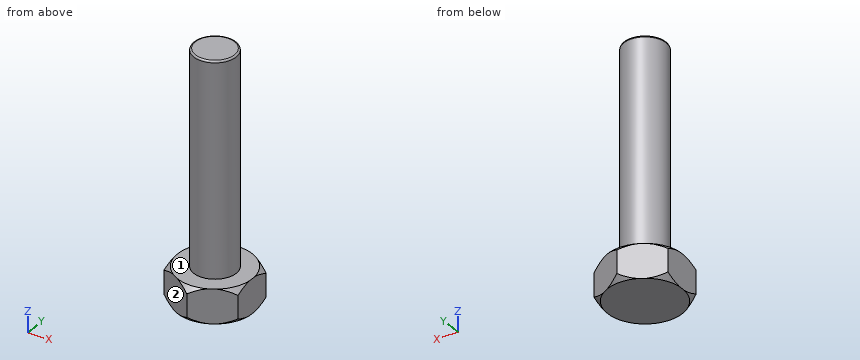
from build123d import *

# Parameters (mm, degrees)
EXTRUDE_1_DEPTH = 3.2
SKETCH_2_R      = 2
EXTRUDE_2_DEPTH = 20
FILLET_1_R      = 0.16


with BuildPart() as part:
    # 草图1 → 凸台-拉伸1 (new body)
    with BuildSketch(Plane.XY):
        Polygon((0, 4.041451884), (-3.5, 2.020725942), (-3.5, -2.020725942), (0, -4.041451884), (3.5, -2.020725942), (3.5, 2.020725942), align=None)
    extrude(amount=-EXTRUDE_1_DEPTH)

    # 草图2 → 凸台-拉伸2 (add)
    with BuildSketch(Plane.XY):
        Circle(SKETCH_2_R)
    extrude(amount=EXTRUDE_2_DEPTH)

    # 圆角1
    fillet_1_edges = [part.edges().sort_by_distance(p)[0] for p in [
        (-2, 0, 20),
    ]]
    fillet(fillet_1_edges, radius=FILLET_1_R)

    # 草图3 → 切除-旋转1 (revolve, cut)
    with BuildSketch(Plane(origin=(0, 0, 0), x_dir=(0, 0, -1), z_dir=(1, 0, 0))):
        Polygon((0.523, 4.041451884), (0, 3.518451884), (0, 4.041451884), align=None)
        Polygon((3.2, 4.041451884), (3.2, 3.518451884), (2.677, 4.041451884), align=None)
    revolve(axis=Axis((0, 0, 0), (0, 0, 1)), mode=Mode.SUBTRACT)


solid = part.part
Verification items for the finished model (mm, model axes). Face numbers are marked on the shaded views. A direction names the side the tool comes from. Coordinates: 2 decimals unless noted, no trailing zeros. Order: outer loops, then holes, each group sorted by start corner. A loop starts at its lowest first (then second) coordinate and runs counter-clockwise, first axis right, second up.
1. Sectioned sample at B-B, the plane z = 9.75. Record the cut outline in (x, y).
Results found:
outline: circle Ø4 at (0, 0)
2. Scan lines: line 1 (Z direction, x = -0.5, y = 2.5); line 2 (Y direction, x = -1.75, z = 19); line 3 (X direction, y = -1.5, z = 14.5). Record each from-to range of solid material in increasing order.
Results found:
line 1: z = -3.2 to 0
line 2: y = -0.97 to 0.97
line 3: x = -1.32 to 1.32
3. Sectioned sample at A-A, the plane y = 0. Record the cut outline in (x, z).
Results found:
outline: (-3.5, -3.2) - (3.5, -3.2) - (3.5, 0) - (2, 0) - (2, 19.84) arc R0.16 ccw to (1.84, 20) - (-1.84, 20) arc R0.16 ccw to (-2, 19.84) - (-2, 0) - (-3.5, 0) - close
4. Go/stop test with flat-tipped pins: pin 1 Ø1.5 at (x, z) = (-1.5, 7) entering from -Y; pin 2 Ø1.5 at (y, z) = (2.5, 15) entering from -X; pin 3 Ø4 at (y, z) = (-1, 2.5) entering from -X. Record where each tip stops, or that it passes through.
Results found:
pin 1: stops at y = -1.85
pin 2: stops at x = -0.97
pin 3: stops at x = -2
5. Set-up check for the marked faces 1 and 2: record each of +Z, -Z, +X, -X, +Y, -Y from which the full face is reachable in a straight line by a thin tool's end or side.
Results found:
face 1: +Z
face 2: +Z, -Z, -X, -Y
